Build history of the part. All positions in model axes, mm. Face numbers are marked on the shaded views. A direction names the side the tool comes from. Round coordinates to 2 decimals unless told otherwise and drop trailing zeros. Order: outer loops, then holes, each group sorted by start corner. A loop starts at its lowest first (then second) coordinate and runs counter-clockwise, first axis right, second up. Notation, with made-up numbers: (16.5, -15.75) -> (35.5, -15.75) arc R14 cw to (35.5, -9.75) -> close; hole circle Ø11 at (49.25, 40.5). An arc over 180 degrees is marked (long way). Use a Markdown table: item, result. Add a question column.
Item 1: Slice it at C-C, the plane z = 0. Give the cut face in (x, y).
Item 2: Slice it at B-B, the plane y = 108.7. Give the cut face in (x, z).
Item 3: Pin check, flat tips, straight feed: pin 1 (10 mm diameter, centred on x = -12, z = 0.5, fed in from -Y); pin 2 (2 mm diameter, centred on y = 2, z = 16, fed in from -X); pin 3 (11 mm diameter, centred on x = -8, y = 41, fed in from +Z); pin 4 (1.5 mm diameter, centred on y = 105, z = -4, fed in from -X). Stop position of each tip, or through.
Item 4: Slice it at A-A, the plane x = 15. Give the cut face in (y, z).
Item 5: Probe L1, parallel to Y at x = -2.5, z = -0.5; L2, parallel to Z at x = 0, y = 4.75; L3, parallel to Z at x = -15, y = 2. List the from-to ranges inside material, lowest first.
Item 6: 3-axis set-ups, long thin cutter, end or side, ignore diameter. For the marked faces 1 and 2: which of +Z, -Z, +X, -X, +Y, -Y reach the whole face in a straight line?
Item 7: Slice it at D-D, the plane y = 52.5. Give the cut face in (x, z).
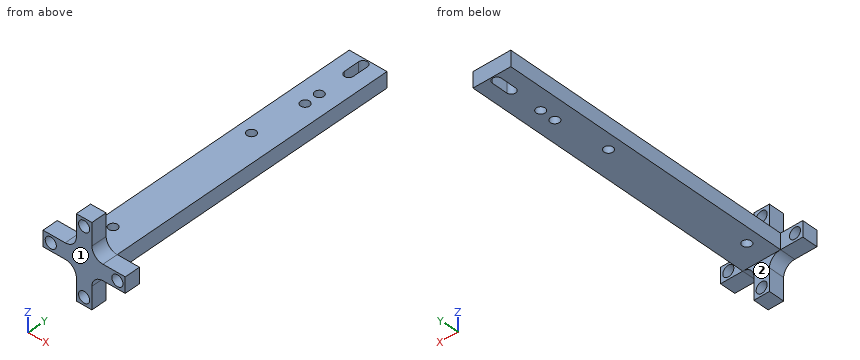
from build123d import *

# Parameters (mm, degrees)
SKETCH1_W           = 17
SKETCH1_H           = 7
BOSS_EXTRUDE1_DEPTH = 139.7
SKETCH2_R           = 2.5
BOSS_EXTRUDE2_DEPTH = 7
FILLET1_R           = 5
SKETCH3_R           = 2
CUT_EXTRUDE1_DEPTH  = 7
SKETCH4_R           = 2
CUT_EXTRUDE2_DEPTH  = 7


with BuildPart() as part:
    # Sketch1 → Boss-Extrude1 (new body)
    with BuildSketch(Plane(origin=(0, 0, 0), x_dir=(1, 0, 0), z_dir=(0, 1, 0))):
        Rectangle(SKETCH1_W, SKETCH1_H)
    extrude(amount=BOSS_EXTRUDE1_DEPTH)

    # Sketch2 → Boss-Extrude2 (add)
    with BuildSketch(Plane(origin=(0, 0, 0), x_dir=(1, 0, 0), z_dir=(0, 1, 0))):
        Polygon((-3.5, 3.5), (-3.5, 18.5), (3.5, 18.5), (3.5, 3.5), (8.5, 3.5), (18.5, 3.5), (18.5, -3.5), (8.5, -3.5), (3.5, -3.5), (3.5, -18.5), (-3.5, -18.5), (-3.5, -3.5), (-8.5, -3.5), (-18.5, -3.5), (-18.5, 3.5), (-8.5, 3.5), align=None)
        with Locations((0, 15)):
            Circle(SKETCH2_R, mode=Mode.SUBTRACT)
        with Locations((15, 0)):
            Circle(SKETCH2_R, mode=Mode.SUBTRACT)
        with Locations((0, -15)):
            Circle(SKETCH2_R, mode=Mode.SUBTRACT)
        with Locations((-15, 0)):
            Circle(SKETCH2_R, mode=Mode.SUBTRACT)
    extrude(amount=BOSS_EXTRUDE2_DEPTH)

    # Fillet1
    fillet1_edges = [part.edges().sort_by_distance(p)[0] for p in [
        (-3.5, 3.5, 3.5),
        (3.5, 3.5, 3.5),
        (3.5, 3.5, -3.5),
        (-3.5, 3.5, -3.5),
    ]]
    fillet(fillet1_edges, radius=FILLET1_R)

    # Sketch3 → Cut-Extrude1 (cut)
    with BuildSketch(Plane.XY.offset(3.5)):
        with Locations((-2.5, 85.072)):
            Circle(SKETCH3_R)
        with Locations((-2.5, 17)):
            Circle(SKETCH3_R)
    extrude(amount=-CUT_EXTRUDE1_DEPTH, mode=Mode.SUBTRACT)

    # Sketch4 → Cut-Extrude2 (cut)
    with BuildSketch(Plane.XY.offset(3.5)):
        with Locations((0, 115.7)):
            Circle(SKETCH4_R)
        with Locations((0, 108.7)):
            Circle(SKETCH4_R)
        with BuildLine():
            Line((2, 137.2), (2, 130.2))
            ThreePointArc((2, 130.2), (0, 128.2), (-2, 130.2))
            Line((-2, 130.2), (-2, 137.2))
            ThreePointArc((-2, 137.2), (0, 139.2), (2, 137.2))
        make_face()
    extrude(amount=-CUT_EXTRUDE2_DEPTH, mode=Mode.SUBTRACT)


solid = part.part
Check sheet entries:
| question | item | result |
|---|---|---|
| 1 | outline | (-18.5, 0) -> (-17.5, 0) -> (-17.5, 7) -> (-18.5, 7) -> close; (-12.5, 0) -> (12.5, 0) -> (12.5, 7) -> (8.5, 7) -> (8.5, 139.7) -> (-8.5, 139.7) -> (-8.5, 7) -> (-12.5, 7) -> close; (17.5, 0) -> (18.5, 0) -> (18.5, 7) -> (17.5, 7) -> close; hole circle Ø4 at (-2.5, 17); hole circle Ø4 at (-2.5, 85.07); hole circle Ø4 at (0, 108.7); hole circle Ø4 at (0, 115.7); hole (-2, 130.2) arc R2 ccw to (2, 130.2) -> (2, 137.2) arc R2 ccw to (-2, 137.2) -> close |
| 2 | outline | (-8.5, -3.5) -> (-2, -3.5) -> (-2, 3.5) -> (-8.5, 3.5) -> close; (2, -3.5) -> (8.5, -3.5) -> (8.5, 3.5) -> (2, 3.5) -> close |
| 3 | pin 1 | y = 0 |
| 3 | pin 2 | x = -3.5 |
| 3 | pin 3 | z = 3.5 |
| 3 | pin 4 | x = -8.5 |
| 4 | outline | (0, -3.5) -> (7, -3.5) -> (7, -2.5) -> (0, -2.5) -> close; (0, 2.5) -> (7, 2.5) -> (7, 3.5) -> (0, 3.5) -> close |
| 5 | L1 | 0 to 15, 19 to 83.07, 87.07 to 139.7 |
| 5 | L2 | -18.5 to -17.5, -12.5 to 12.5, 17.5 to 18.5 |
| 5 | L3 | -3.5 to -2.5, 2.5 to 3.5 |
| 6 | face 1 | +Z, -Z, +X, -X, -Y |
| 6 | face 2 | -Z, +X, -X, +Y |
| 7 | outline | (-8.5, -3.5) -> (8.5, -3.5) -> (8.5, 3.5) -> (-8.5, 3.5) -> close |
